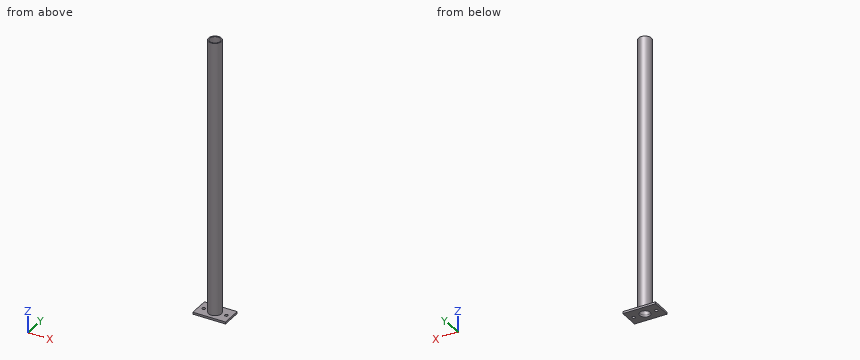
Autodesk Inventor part; units mm, degrees
ref_plane "YZ Plane" through (0, 0, 0) normal (1, 0, 0) x (0, 1, 0)
ref_plane "XZ Plane" through (0, 0, 0) normal (0, 1, 0) x (-1, 0, 0)
ref_plane "XY Plane" through (0, 0, 0) normal (0, 0, 1) x (1, 0, 0)
sketch "Boceto1" plane through (0, 0, 0) normal (0, 0, 1) x (1, 0, 0)
  circle A0 centre (0, 0) radius 25.4
  circle A1 centre (0, 0) radius 20.9
  dimension "d0" = 50.8
  dimension "d1" = 41.8
extrude "Extrusión1" add sketch "Boceto1" along normal blind 1095
sketch "Boceto2" plane through (0, 0, 0) normal (0, 0, -1) x (-1, 0, 0)
  line L0 (-65, -40) -> (65, -40)
  line L1 (65, -40) -> (65, 40)
  line L2 (65, 40) -> (-65, 40)
  line L3 (-65, 40) -> (-65, -40)
  line L4 (-65, -40) -> (65, 40) construction
  line L5 (65, -40) -> (-65, 40) construction
  line L6 (-65, 0) -> (-25.4, 0)
  circle A0 centre (0, 0) radius 25.4
  circle A1 centre (-45.2, 0) radius 6.5
  line L7 (25.4, 0) -> (65, 0)
  circle A2 centre (45.2, 0) radius 6.5
  circle A3 centre (0, 0) radius 25.4
  circle A4 centre (0, 0) radius 20.9
  dimension "d4" = 130
  dimension "d5" = 80
  dimension "d6" = 13
  dimension "d7" = 13
extrude "Extrusión2" add sketch "Boceto2" along normal blind 8 contours L3 L6 A1 A0 L7 A2 L1 L0 | L3 L2 L1 L7 A2 A0 L6 A1 | A0
properties part number "tubo_principal"
Read the model definition and answer for the solid it produces. Units are mm, in the model's axes. Give positions to 0.01 mm unless a question says otherwise; leave off trailing zeros. Order: outer loops, then holes, each group sorted by start corner. A loop starts at its lowest first (then second) coordinate and runs counter-clockwise, first axis right, second up.
(1) Straight lines are drawn through the part: L1, parallel to X at y = 0, z = -3.25; L2, parallel to Y at x = 0, z = 772.5; L3, parallel to Z at x = 31.5, y = -1. For each, find the intervals that lie inside material, in ascending order.
(2) Find section B-B (z = 403). Give the vertices of the cut face in (x, y), plus the area to 3 significant figures.
(3) Given pin 1 (12 mm diameter, centred on y = 4.5, z = 419, fed in from -X); pin 2 (4 mm diameter, centred on y = -15, z = 643, fed in from +X); pin 3 (10 mm diameter, centred on x = 28.5, z = 449, fed in from -Y), each flat-ended and moving along its own axis, determine where each tip first touches the part or whether it passes through.
(4) Find section A-A (x = -1). Give the vertices of the cut face in (y, z).
Result sheet:
1. L1: x = -65 to -51.7, -38.7 to -20.9, 20.9 to 38.7, 51.7 to 65
1. L2: y = -25.4 to -20.9, 20.9 to 25.4
1. L3: z = -8 to 0
2. outline: circle Ø50.8 at (0, 0); hole circle Ø41.8 at (0, 0)
2. area: 655 mm2
3. pin 1: stops at x = -25.4
3. pin 2: stops at x = 21.82
3. pin 3: stops at y = -9.64
4. outline: (-40, -8) - (-20.88, -8) - (-20.88, 1095) - (-25.38, 1095) - (-25.38, 0) - (-40, 0) - close; (20.88, -8) - (40, -8) - (40, 0) - (25.38, 0) - (25.38, 1095) - (20.88, 1095) - close
